Part print with two shaded views. Sizes in mm from the minimum x, y, z corner. A direction names the side the tool comes from. Give positions to 0.01 mm unless a question says otherwise; leave off trailing zeros. Write each loop counter-clockwise with the first axis right and the second up, starting at its lowest first coordinate (ties: lowest second). Pieces come first, ordered by that corner, then holes. Notation, with made-up numbers: (3.5, 41) - (41.5, 41) arc R10 cw to (41.5, 58) - close; hole circle Ø2 at (-30.75, 43.5). An arc over 180 degrees is marked (long way). One line per item, written item: value. Start each with the question number.
(1) Cut at A-A, the plane x = 35. List the corners of the cut face in (y, z), and give its area (3 significant figures).
(2) 3-axis set-ups, long thin cutter, end or side, ignore diameter. For the marked faces 5, 6, 7, 8 and 9: which of +Z, -Z, +X, -X, +Y, -Y reach the whole face in a straight line?
(3) Mould opens along Z. For the marked faces 1, 2, 3 and 4 say: pulls with the +Z half, pulls with the -Z half, needs draft (parallel to the pull), parting line crosses it, or undercut.
(4) Probe L1, parallel to Y at x = 35, z = 8.1; L2, parallel to Y at x = 38, z = 13.25; L3, parallel to X at y = 5.5, z = 6.5. List the from-to ranges inside material, lowest first.
(5) Cut at D-D, the plane z = 2.5. List the corners of the cut face in (x, y), and give its area (3 significant figures).
(6) Drop flat-ended pins along their axis: P1, Ø8, axis at y = 16, z = 10.5, coming from the +X side; P2, Ø5.5, axis at x = 10.5, z = 5.5, coming from the +Y side; P3, Ø5, axis at x = 35.5, y = 19.5, coming from the +Z side. Give the stop position or say it passes through.
(7) Cut at C-C, the plane y = 5. List the corners of the cut face in (x, z), and give its area (3 significant figures).
(8) Cut at B-B, the plane z = 9. List the corners of the cut face in (x, y).
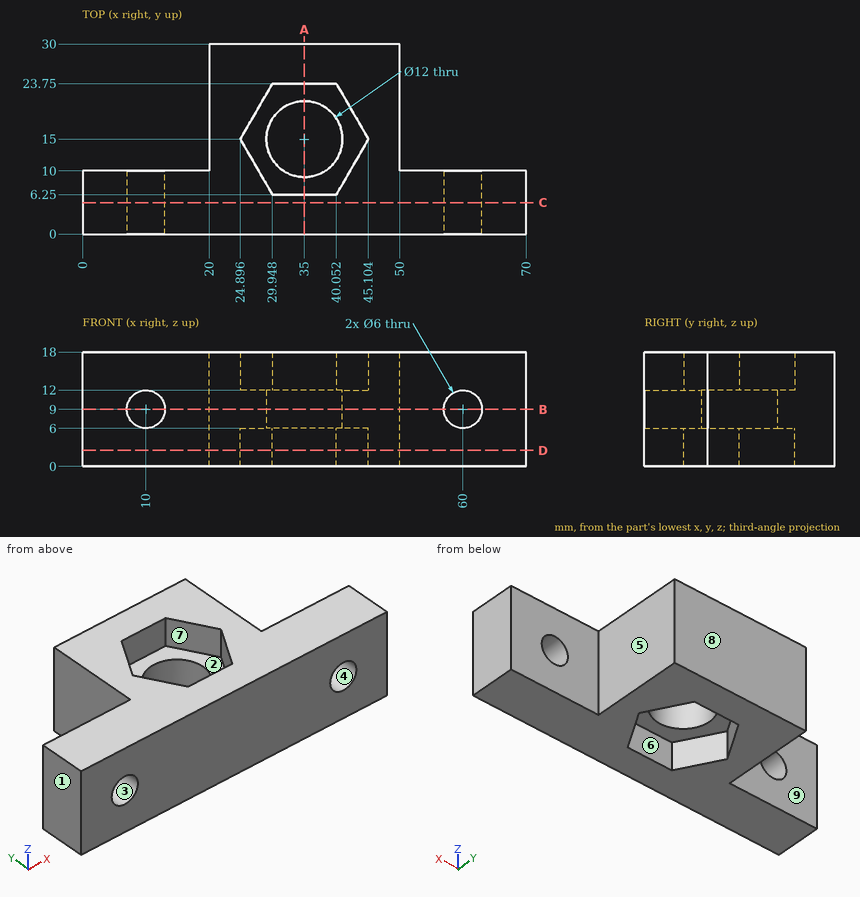
Answers follow:
1. outline: (0, 0) - (6.25, 0) - (6.25, 6) - (9, 6) - (9, 12) - (6.25, 12) - (6.25, 18) - (0, 18) - close; (21, 6) - (23.75, 6) - (23.75, 0) - (30, 0) - (30, 18) - (23.75, 18) - (23.75, 12) - (21, 12) - close
1. area: 258 mm²
2. face 5: +Z, -Z, +X, +Y
2. face 6: -Z
2. face 7: +Z
2. face 8: +Z, -Z, +X, -X, +Y
2. face 9: +Z, -Z, -X, +Y
3. face 1: needs draft
3. face 2: pulls with the +Z half
3. face 3: undercut
3. face 4: undercut
4. L1: y = 0 to 9, 21 to 30
4. L2: y = 0 to 6.25, 23.75 to 30
4. L3: x = 0 to 8.34, 11.66 to 58.34, 61.66 to 70
5. outline: (0, 0) - (70, 0) - (70, 10) - (50, 10) - (50, 30) - (20, 30) - (20, 10) - (0, 10) - close; hole (24.9, 15) - (29.95, 6.25) - (40.05, 6.25) - (45.1, 15) - (40.05, 23.75) - (29.95, 23.75) - close
5. area: 1,030 mm²
6. P1: stops at x = 50
6. P2: stops at y = 10
6. P3: stops at z = 12
7. outline: (0, 0) - (70, 0) - (70, 18) - (0, 18) - close; hole circle Ø6 at (10, 9); hole circle Ø6 at (60, 9)
7. area: 1,200 mm²
8. outline: (0, 0) - (7, 0) - (7, 10) - (0, 10) - close; (13, 0) - (57, 0) - (57, 10) - (50, 10) - (50, 30) - (20, 30) - (20, 10) - (13, 10) - close; (63, 0) - (70, 0) - (70, 10) - (63, 10) - close; hole circle Ø12 at (35, 15)
